from build123d import *

# Parameters (mm, degrees)
BOSS_EXTRUDE1_DEPTH = 5.334


with BuildPart() as part:
    # Sketch1 → Boss-Extrude1 (new body)
    with BuildSketch(Plane.XY):
        with BuildLine():
            ThreePointArc((42.977057526, 61.379780274), (0, 74.93), (-42.977057526, 61.379780274))
            ThreePointArc((-42.977057526, 61.379780274), (-42.944185328, 52.882612065), (-34.518993211, 51.778489817))
            ThreePointArc((-34.518993211, 51.778489817), (0, 62.23), (34.518993211, 51.778489817))
            ThreePointArc((34.518993211, 51.778489817), (42.944185328, 52.882612065), (42.977057526, 61.379780274))
        make_face()
        Polygon((-38.1, 60.816174209), (-41.275, 58.983087105), (-41.275, 55.316912895), (-38.1, 53.483825791), (-34.925, 55.316912895), (-34.925, 58.983087105), align=None, mode=Mode.SUBTRACT)
        Polygon((38.1, 60.816174209), (34.925, 58.983087105), (34.925, 55.316912895), (38.1, 53.483825791), (41.275, 55.316912895), (41.275, 58.983087105), align=None, mode=Mode.SUBTRACT)
    extrude(amount=BOSS_EXTRUDE1_DEPTH)


solid = part.part
Part model, mm, in its own coordinate system. A direction names the side the tool comes from. Coordinates: 2 decimals unless noted, no trailing zeros. Loops run counter-clockwise (first coordinate to the right, second up) from the corner with the lowest first, then second, coordinate; pieces in that order, holes last. Notation, with made-up numbers: M -23.75,-1 L 21.25,-1 A25 cw 21.25,27 Z; hole C 80.5,-21 d7. An arc over 180 degrees is marked long. Use a Markdown table: item, result. Add a question column.
Q1. Mould opens along X. For faces 3 (the cylindrical face through (0.641, 74.927, 2.63)), 4 (the flat face through (-36.49, 59.887, 2.63)), 5 (the flat face through (-1, 66, 0)), 6 (the flat face through (-39.67, 59.91, 2.63)) say: +X half, -X half, draft (parallel to the pull), parting line (faces both ways), or undercut.
Q2. Cut at C-C (y = 60). Write the cut outline in (x, z).
Q3. Probe L1, parallel to X at y = 57.25, z = 2.95 (3 decimals); L2, parallel to X at y = 56, z = 5 (1 decimal); L3, parallel to X at y = 52.75, z = 4.2. List the from-to ranges inside material, lowest first.
Q4. Cut at D-D (x = 1). Write the cut outline in (y, z), and give its area (3 significant figures).
Q5. Which spindle directions (+Z, -Z, +X, -X, +Y, -Y) get a long thin tool onto all of the face, cutting with end or side? Do faces 1 (the flat face through (36.53, 59.91, 2.63)), 2 (the cylindrical face through (-0.512, 62.228, 2.63)). Say none if no direction does.
Q6. Pin check, flat tip, straight feed: P1, Ø3, axis at y = 67, z = 2, coming from the -X side. Stop position of the tip, or through.
Q7. Cut at A-A (z = 1.4). Give the number of separate pieces and of enclosed holes in the cut face, and give its area (3 significant figures).
Q8. Cut at B-B (y = 56.5). Write the cut outline in (x, z) (3 decimals).
Worked out:
| question | item | result |
|---|---|---|
| 1 | face 3 | parting line |
| 1 | face 4 | undercut |
| 1 | face 5 | draft |
| 1 | face 6 | undercut |
| 2 | outline | M -43.89,0 L -39.51,0 L -39.51,5.33 L -43.89,5.33 Z; M -36.69,0 L -16.51,0 L -16.51,5.33 L -36.69,5.33 Z; M 16.51,0 L 36.69,0 L 36.69,5.33 L 16.51,5.33 Z; M 39.51,0 L 43.89,0 L 43.89,5.33 L 39.51,5.33 Z |
| 3 | L1 | x = -44.555 to -41.275, -34.925 to -24.393, 24.393 to 34.925, 41.275 to 44.555 |
| 3 | L2 | x = -44.5 to -41.3, -34.9 to -27.1, 27.1 to 34.9, 41.3 to 44.5 |
| 3 | L3 | x = -42.82 to -33.02, 33.02 to 42.82 |
| 4 | outline | M 62.22,0 L 74.92,0 L 74.92,5.33 L 62.22,5.33 Z |
| 4 | area | 67.7 mm2 |
| 5 | face 1 | +Z, -Z |
| 5 | face 2 | +Z, -Z, -Y |
| 6 | P1 | stops at x = -36.39 |
| 7 | separate pieces | 1 |
| 7 | enclosed holes | 2 |
| 7 | area | 1,080 mm2 |
| 8 | outline | M -44.523,0 L -41.275,0 L -41.275,5.334 L -44.523,5.334 Z; M -34.925,0 L -26.083,0 L -26.083,5.334 L -34.925,5.334 Z; M 26.083,0 L 34.925,0 L 34.925,5.334 L 26.083,5.334 Z; M 41.275,0 L 44.523,0 L 44.523,5.334 L 41.275,5.334 Z |
